Here's how the part is built. I have some questions about the finished solid (model axes, mm). A direction names the side the tool comes from. Give positions to 0.01 mm unless a question says otherwise; leave off trailing zeros. Loops run counter-clockwise (first coordinate to the right, second up) from the corner with the lowest first, then second, coordinate; pieces in that order, holes last. Notation, with made-up numbers: (4.5, 25) - (55.5, 25) arc R17 cw to (55.5, 57) - close; hole circle Ø6 at (52.25, 35.5). An arc over 180 degrees is marked (long way). Return JSON: item names as keys, results as strings. Group by question number.
(1) If we section it at B-B (y = 63.5): Please give me the cut outline in (x, z), then the cut area to 3 significant figures.
(2) If we section it at A-A (x = -24): Please give me the cut outline in (y, z), then the cut area to 3 significant figures.
(3) On a 3-axis mill with a long thin cutter (end or side, diameter ignored), from which of +Z, -Z, +X, -X, +Y, -Y can I reach the whole of each face in a straight line? I mean faces 1 (the cylindrical face through (-27.438, 59.181, 0.042)), 2 (the flat face through (26, 75, 0)), 3 (the cylindrical face through (13.01, 12.85, 0.04)). Say none if no direction works.
(4) I need wall thicknesses on probe 1 along Y at (x, z) = (-18.5, 1.45); probe 2 along Y at (x, z) = (-22, 0.75); probe 3 along X at (y, z) = (56, -0.7). Which ranges of each line are inside material? Lowest first, please. Write a range as [from, to].
(5) If we section it at D-D (x = 0): Please give me the cut outline in (y, z), then the cut area to 3 significant figures.
(6) If we section it at C-C (z = 0): Please give me the cut outline in (x, y), then the cut area to 3 significant figures.
(7) For P1, Ø1, axis at x = -6.5, z = 0.5, coming from the +Y side; P2, Ø3, axis at y = 28, z = 1, coming from the -X side, each with a flat end and sliding along its axis, tell me the tip position at first contact or that it passes through.
```python
from build123d import *

# Parameters (mm, degrees)
BOSS_EXTRU_1_DEPTH = 3


with BuildPart() as part:
    # Esquisse1 → Boss.-Extru.1 (new body, symmetric)
    with BuildSketch(Plane.XY):
        with BuildLine():
            Line((-40, 0), (40, 0))
            Line((40, 0), (40, 10))
            Line((40, 10), (20, 10))
            ThreePointArc((20, 10), (12.928932188, 12.928932188), (10, 20))
            Line((10, 20), (10, 31.876730806))
            ThreePointArc((10, 31.876730806), (12.144695993, 40.88717579), (18.118811881, 47.965154249))
            ThreePointArc((18.118811881, 47.965154249), (27.348830005, 58.998463148), (30.495305887, 73.035087719))
            ThreePointArc((30.495305887, 73.035087719), (29.897366986, 74.426565007), (28.495613698, 75))
            Line((28.495613698, 75), (22.494443758, 75))
            ThreePointArc((22.494443758, 75), (21.064603052, 74.398411798), (20.494937647, 72.955555556))
            ThreePointArc((20.494937647, 72.955555556), (0, 52), (-20.494937647, 72.955555556))
            ThreePointArc((-20.494937647, 72.955555556), (-21.064603052, 74.398411798), (-22.494443758, 75))
            Line((-22.494443758, 75), (-28.495613698, 75))
            ThreePointArc((-28.495613698, 75), (-29.897366986, 74.426565007), (-30.495305887, 73.035087719))
            ThreePointArc((-30.495305887, 73.035087719), (-27.348830005, 58.998463148), (-18.118811881, 47.965154249))
            ThreePointArc((-18.118811881, 47.965154249), (-12.144695993, 40.88717579), (-10, 31.876730806))
            Line((-10, 31.876730806), (-10, 20))
            ThreePointArc((-10, 20), (-12.928932188, 12.928932188), (-20, 10))
            Line((-20, 10), (-40, 10))
            Line((-40, 10), (-40, 0))
        make_face()
    extrude(amount=BOSS_EXTRU_1_DEPTH, both=True)


solid = part.part
```
Values:
{
 "1": {"outline": "(-29.14, -3) - (-18.42, -3) - (-18.42, 3) - (-29.14, 3) - close; (18.42, -3) - (29.14, -3) - (29.14, 3) - (18.42, 3) - close", "area": "129 mm2"},
 "2": {"outline": "(0, -3) - (10, -3) - (10, 3) - (0, 3) - close; (53.68, -3) - (75, -3) - (75, 3) - (53.68, 3) - close", "area": "188 mm2"},
 "3": {"face 1": "+Z, -Z, -X", "face 2": "+Z, -Z, +X, -X, +Y", "face 3": "+Z, -Z, +X"},
 "4": {"probe 1": "[0, 10.11], [48.25, 63.67]", "probe 2": "[0, 10], [51.38, 74.94]", "probe 3": "[-25.65, -12.17], [12.17, 25.65]"},
 "5": {"outline": "(0, -3) - (52, -3) - (52, 3) - (0, 3) - close", "area": "312 mm2"},
 "6": {"outline": "(-40, 0) - (40, 0) - (40, 10) - (20, 10) arc R10 cw to (10, 20) - (10, 31.88) arc R20 cw to (18.12, 47.97) arc R30.5 ccw to (30.5, 73.04) arc R2 ccw to (28.5, 75) - (22.49, 75) arc R2 ccw to (20.49, 72.96) arc R20.5 cw (long way) to (-20.49, 72.96) arc R2 ccw to (-22.49, 75) - (-28.5, 75) arc R2 ccw to (-30.5, 73.04) arc R30.5 ccw to (-18.12, 47.97) arc R20 cw to (-10, 31.88) - (-10, 20) arc R10 cw to (-20, 10) - (-40, 10) - close", "area": "2,380 mm2"},
 "7": {"P1": "y = 53.23", "P2": "x = -10"}
}
